from build123d import *

# Parameters (mm, degrees)
SZKIC1_W                    = 104
SZKIC1_H                    = 118.94
DODANIE_WYCI_GNI_CIE1_DEPTH = 2
SZKIC2_W                    = 53
SZKIC2_H                    = 1.6
SZKIC2_H_2                  = 6.407346329
WYTNIJ_WYCI_GNI_CIE2_DEPTH  = 2
SZKIC4_W                    = 2
SZKIC4_H                    = 118.94
DODANIE_WYCI_GNI_CIE2_DEPTH = 2
SZKIC5_R                    = 1.6
WYTNIJ_WYCI_GNI_CIE3_DEPTH  = 2
ZAOKR_GLENIE1_R             = 2
SZKIC6_R                    = 6.5
SZKIC6_R_2                  = 7.5
WYTNIJ_WYCI_GNI_CIE4_DEPTH  = 12
WYTNIJ_WYCI_GNI_CIE5_DEPTH  = 12
ZAOKR_GLENIE2_R             = 2


with BuildPart() as part:
    # Szkic1 → Dodanie-wyciągnięcie1 (new body)
    with BuildSketch(Plane.XY):
        with Locations((56, 59.47)):
            Rectangle(SZKIC1_W, SZKIC1_H)
    extrude(amount=DODANIE_WYCI_GNI_CIE1_DEPTH)

    # Szkic2 → Wytnij-wyciągnięcie2 (cut)
    with BuildSketch(Plane(origin=(0, 0, 0), x_dir=(-1, 0, 0), z_dir=(0, 0, -1))):
        with Locations((-46.5, 8.8)):
            Rectangle(SZKIC2_W, SZKIC2_H)
        with Locations((-46.5, 12.803673165)):
            Rectangle(SZKIC2_W, SZKIC2_H_2)
    extrude(amount=-WYTNIJ_WYCI_GNI_CIE2_DEPTH, mode=Mode.SUBTRACT)

    # Szkic4 → Dodanie-wyciągnięcie2 (add)
    with BuildSketch(Plane(origin=(0, 0, 0), x_dir=(-1, 0, 0), z_dir=(0, 0, -1))):
        with Locations((-3, 59.47)):
            Rectangle(SZKIC4_W, SZKIC4_H)
        with Locations((-109, 59.47)):
            Rectangle(SZKIC4_W, SZKIC4_H)
    extrude(amount=-DODANIE_WYCI_GNI_CIE2_DEPTH)

    # Szkic5 → Wytnij-wyciągnięcie3 (cut)
    with BuildSketch(Plane.XY.offset(2)):
        with Locations((8, 12)):
            Circle(SZKIC5_R)
        with Locations((104, 12)):
            Circle(SZKIC5_R)
        with Locations((8, 106.94)):
            Circle(SZKIC5_R)
        with Locations((104, 106.94)):
            Circle(SZKIC5_R)
    extrude(amount=-WYTNIJ_WYCI_GNI_CIE3_DEPTH, mode=Mode.SUBTRACT)

    # Zaokrąglenie1
    zaokr_glenie1_edges = [part.edges().sort_by_distance(p)[0] for p in [
        (110, 59.47, 2),
        (2, 59.47, 2),
    ]]
    fillet(zaokr_glenie1_edges, radius=ZAOKR_GLENIE1_R - 0.0001)  # a hair under: the kernel refuses the full size

    # Szkic6 → Wytnij-wyciągnięcie4 (cut)
    with BuildSketch(Plane.XY.offset(2)):
        with Locations((72, 66)):
            Circle(SZKIC6_R)
        with Locations((40, 66)):
            Circle(SZKIC6_R_2)
    extrude(amount=-WYTNIJ_WYCI_GNI_CIE4_DEPTH, mode=Mode.SUBTRACT)

    # Szkic7 → Wytnij-wyciągnięcie5 (cut)
    with BuildSketch(Plane.XY.offset(2)):
        Polygon((56, 55), (98, 55), (98, 40), (14, 40), (14, 55), align=None)
    extrude(amount=-WYTNIJ_WYCI_GNI_CIE5_DEPTH, mode=Mode.SUBTRACT)

    # Zaokrąglenie2
    zaokr_glenie2_edges = [part.edges().sort_by_distance(p)[0] for p in [
        (14, 55, 1),
        (98, 55, 1),
        (98, 40, 1),
        (14, 40, 1),
    ]]
    fillet(zaokr_glenie2_edges, radius=ZAOKR_GLENIE2_R)


solid = part.part
Part model, mm, in its own coordinate system. Round coordinates to 2 decimals unless told otherwise and drop trailing zeros. Write each loop counter-clockwise with the first axis right and the second up, starting at its lowest first coordinate (ties: lowest second). Pieces come first, ordered by that corner, then holes. Notation, with made-up numbers: M 67.5,-12.5 L 125.5,-12.5 A16 ccw 125.5,0.5 Z; hole C 41.5,76 d3. An arc over 180 degrees is marked long. Return JSON: item names as keys, results as strings. Group by question number.
(1) Saw through at A-A on x = 8. Write the cut outline in (y, z).
(2) Saw through at C-C on x = 93. Write the cut outline in (y, z), then the cut area to 3 significant figures.
(3) Two-plate mould, pull along X, no slides. Class faces 1 (the face through (7.792, 108.526, 1.014)), 2 (the face through (32.507, 66.33, 1.014)), 3 (the face through (57, 60, 0)): +X half, -X half, draft (parallel to the pull), parting line (faces both ways), or undercut.
(4) Drill centre lines: probe 1 along Y at (x, z) = (8, 1.15); probe 2 along Y at (x, z) = (52.5, 0.35); probe 3 along Y at (x, z) = (40, 1.6). Where is each one in solid material? Low to high.
(5) Saw through at B-B on y = 66. Count the separate pieces of the cut face and the enclosed holes in it, then the cut area to 3 significant figures.
(6) Pin check, flat tips, straight feed: pin 1 Ø0.6 at (y, z) = (13, 0.5) entering from +X; pin 2 Ø1 at (y, z) = (11, 1) entering from -X. Stop position of each tip, or through.
Returned:
{
 "1": {"outline": "M 0,0 L 10.4,0 L 10.4,2 L 0,2 Z; M 13.6,0 L 105.34,0 L 105.34,2 L 13.6,2 Z; M 108.54,0 L 118.94,0 L 118.94,2 L 108.54,2 Z"},
 "2": {"outline": "M 0,0 L 40,0 L 40,2 L 0,2 Z; M 55,0 L 118.94,0 L 118.94,2 L 55,2 Z", "area": "208 mm²"},
 "3": {"face 1": "undercut", "face 2": "undercut", "face 3": "draft"},
 "4": {"probe 1": "0 to 10.4, 13.6 to 105.34, 108.54 to 118.94", "probe 2": "0 to 8, 16.01 to 40, 55 to 118.94", "probe 3": "0 to 8, 16.01 to 40, 55 to 58.5, 73.5 to 118.94"},
 "5": {"separate pieces": "3", "enclosed holes": "0", "area": "158 mm²"},
 "6": {"pin 1": "x = 109.99", "pin 2": "x = 2.06"}
}
